Input: part model. Units: mm. Frame: model coordinates. A direction names the side the tool comes from. Round coordinates to 2 decimals unless told otherwise and drop trailing zeros. Loops run counter-clockwise (first coordinate to the right, second up) from the corner with the lowest first, then second, coordinate; pieces in that order, holes last. Notation, with made-up numbers: M -2.75,21 L 9.25,21 A6 cw 9.25,25 Z; hole C -13.5,13 d8. An arc over 180 degrees is marked long. Put each result on its own line as item: value. Start each with the question number.
1) Section B-B on y = 177.8. Output: boundary loops of the cut face in (x, z) (3 decimals), plus the area to 3 significant figures.
2) Pin query (flat end, axial travel): pin 1 (4 mm diameter, centred on y = 36.5, z = -8.5, fed in from +X). Return the tip coordinate at first contact, or that it passes through.
3) Section C-C on y = 121.5. Output: boundary loops of the cut face in (x, z) (3 decimals).
4) Reachability of faces 1 (the face through (0, 100, 11.43)), 2 (the face through (-7.615, 152.819, 12.056)), 3 (the face through (-12.074, 78.877, 1.707)) from +Z, -Z, +X, -X, +Y, -Y: full face, straight path, thin tool, end or side. Return the list, or none.
5) Draft query along Z for faces 4 (the face through (0, 100, -11.43)), 5 (the face through (-12, 0, 0)), 6 (the face through (0, 100, -12.7)), 7 (the face through (0, 100, 12.7)). Return one class per face: +Z half, -Z half, draft (parallel to the pull), parting line (faces both ways), or undercut.
6) Line query: probe 1 along Y at (x, z) = (-11.85, 0) (3 decimals); probe 2 along Z at (x, y) = (-1, 52.5); probe 3 along X at (y, z) = (123, -8). Output: solid intervals per line, ascending.
7) Section A-A on z = 0. Output: boundary loops of the cut face in (x, y) (3 decimals), plus the area to 3 significant figures.
8) Section D-D on y = 147. Output: boundary loops of the cut face in (x, z) (3 decimals).
from build123d import *

# Parameters (mm, degrees)
SKETCH1_W               = 25.4
SKETCH1_H               = 25.4
SKETCH1_W_2             = 22.86
SKETCH1_H_2             = 22.86
BOSS_EXTRUDE1_DEPTH     = 203.2
SKETCH2_W               = 25.4
SKETCH2_H               = 203.2
CUT_EXTRUDE1_DEPTH      = 1.27
SKETCH3_R               = 3.175
CUT_EXTRUDE2_DEPTH      = 1.27
CUT_EXTRUDE3_DEPTH      = 206.174779152
CUT_EXTRUDE3_DEPTH_BACK = 2.54
FILLET10_R              = 1.905


with BuildPart() as part:
    # Sketch1 → Boss-Extrude1 (new body)
    with BuildSketch(Plane(origin=(0, 0, 0), x_dir=(1, 0, 0), z_dir=(0, 1, 0))):
        Rectangle(SKETCH1_W, SKETCH1_H)
        Rectangle(SKETCH1_W_2, SKETCH1_H_2, mode=Mode.SUBTRACT)
    extrude(amount=BOSS_EXTRUDE1_DEPTH)

    # Sketch2 → Cut-Extrude1 (cut)
    with BuildSketch(Plane(origin=(12.7, 0, 0), x_dir=(0, 0, -1), z_dir=(1, 0, 0))):
        with Locations((0, 101.6)):
            Rectangle(SKETCH2_W, SKETCH2_H)
    extrude(amount=-CUT_EXTRUDE1_DEPTH, mode=Mode.SUBTRACT)

    # Sketch3 → Cut-Extrude2 (cut)
    with BuildSketch(Plane.ZY.offset(12.7)):
        with Locations((0, 25.4)):
            Circle(SKETCH3_R)
        with Locations((0, 76.2)):
            Circle(SKETCH3_R)
        with Locations((0, 127)):
            Circle(SKETCH3_R)
        with Locations((0, 177.8)):
            Circle(SKETCH3_R)
    extrude(amount=-CUT_EXTRUDE2_DEPTH, mode=Mode.SUBTRACT)

    # Sketch4 → Cut-Extrude3 (cut, two sides: drawn at the far end of the back side and taken through both)
    with BuildSketch(Plane.XY.offset(12.7).offset(-CUT_EXTRUDE3_DEPTH_BACK)):
        with BuildLine():
            Line((367.709421277, 171.45), (11.43, 171.45))
            ThreePointArc((11.43, 171.45), (-7.62, 152.4), (11.43, 133.35))
            Line((11.43, 133.35), (367.709421277, 133.35))
            Line((367.709421277, 133.35), (1080.268263831, 133.35))
            Line((1080.268263831, 133.35), (1080.268263831, 171.45))
            Line((1080.268263831, 171.45), (367.709421277, 171.45))
        make_face()
    extrude(amount=CUT_EXTRUDE3_DEPTH + CUT_EXTRUDE3_DEPTH_BACK, mode=Mode.SUBTRACT)

    # Fillet10
    fillet10_edges = [part.edges().sort_by_distance(p)[0] for p in [
        (-12.7, 101.6, 12.7),
        (-12.7, 101.6, -12.7),
    ]]
    fillet(fillet10_edges, radius=FILLET10_R)


solid = part.part
Geometry results:
1. outline: M -12.7,-10.795 A1.905 ccw -10.795,-12.7 L 11.43,-12.7 L 11.43,-11.43 L -11.43,-11.43 L -11.43,-3.175 L -12.7,-3.175 Z; M -12.7,3.175 L -11.43,3.175 L -11.43,11.43 L 11.43,11.43 L 11.43,12.7 L -10.795,12.7 A1.905 ccw -12.7,10.795 Z
1. area: 80.7 mm²
2. pin 1: stops at x = -11.43
3. outline: M -12.7,-10.795 A1.905 ccw -10.795,-12.7 L 11.43,-12.7 L 11.43,-11.43 L -11.43,-11.43 L -11.43,11.43 L 11.43,11.43 L 11.43,12.7 L -10.795,12.7 A1.905 ccw -12.7,10.795 Z
4. face 1: +X, +Y, -Y
4. face 2: +Z, +X
4. face 3: +X, -X
5. face 4: undercut
5. face 5: draft
5. face 6: -Z half
5. face 7: +Z half
6. probe 1: y = 0 to 22.225, 28.575 to 73.025, 79.375 to 123.825, 130.175 to 174.625, 180.975 to 203.2
6. probe 2: z = -12.7 to -11.43, 11.43 to 12.7
6. probe 3: x = -12.7 to -11.43
7. outline: M -12.7,0 L -11.43,0 L -11.43,22.225 L -12.7,22.225 Z; M -12.7,28.575 L -11.43,28.575 L -11.43,73.025 L -12.7,73.025 Z; M -12.7,79.375 L -11.43,79.375 L -11.43,123.825 L -12.7,123.825 Z; M -12.7,130.175 L -11.43,130.175 L -11.43,174.625 L -12.7,174.625 Z; M -12.7,180.975 L -11.43,180.975 L -11.43,203.2 L -12.7,203.2 Z
7. area: 226 mm²
8. outline: M -12.7,-10.795 A1.905 ccw -10.795,-12.7 L 11.43,-12.7 L 11.43,-11.43 L -11.43,-11.43 L -11.43,11.43 L -6.839,11.43 L -6.839,12.7 L -10.795,12.7 A1.905 ccw -12.7,10.795 Z
